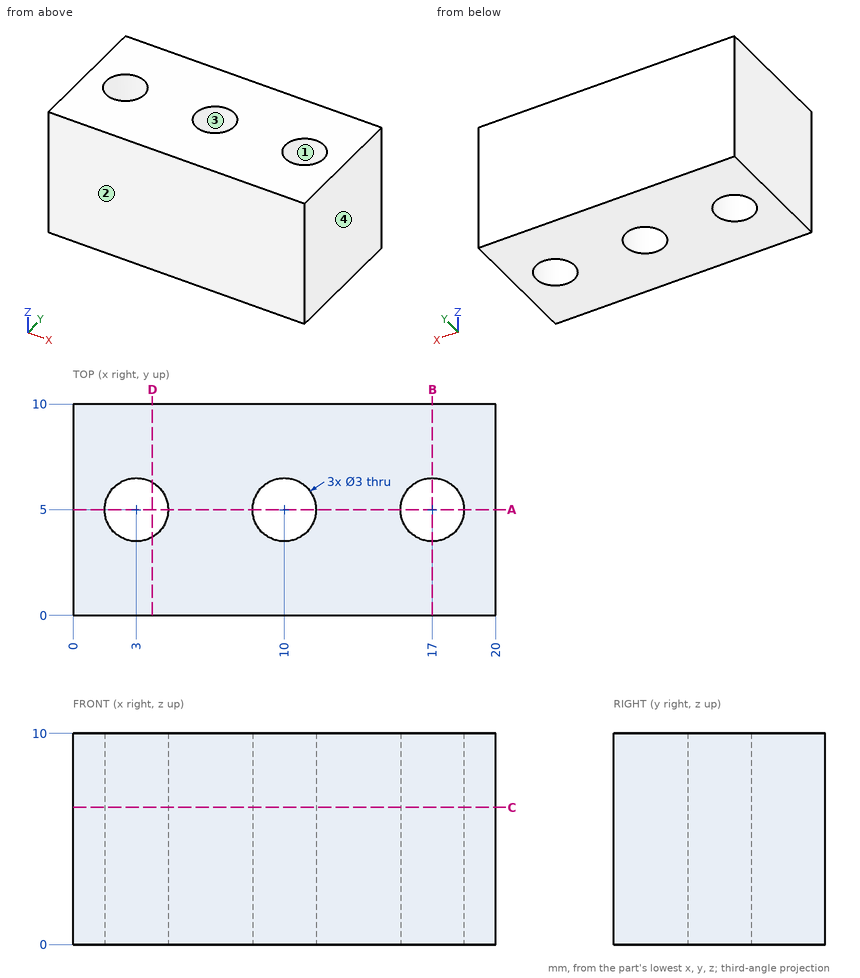
Print and shaded views of the part. All mm, measured from the part's lowest x, y and z. Give positions to 0.01 mm unless a question says otherwise; leave off trailing zeros. Order: outer loops, then holes, each group sorted by start corner. A loop starts at its lowest first (then second) coordinate and runs counter-clockwise, first axis right, second up. Notation, with made-up numbers: (71, 42) - (89, 42) arc R5 ccw to (89, 48) - close; hole circle Ø2 at (-29.75, -4.75). An arc over 180 degrees is marked (long way). Use a Markdown table: item, result.
1) Flat gauge pin, fed straight in: P1, Ø2.5, axis at x = 10, y = 5, coming from the +Z side. Where does the tip first touch, or does it go through?
Checked values:
| item | result |
|---|---|
| P1 | through |
2) Saw through at C-C on z = 6.5. List the corners of the cut face in (x, y), plus the area to 3 significant figures.
Checked values:
| item | result |
|---|---|
| outline | (0, 0) - (20, 0) - (20, 10) - (0, 10) - close; hole circle Ø3 at (3, 5); hole circle Ø3 at (10, 5); hole circle Ø3 at (17, 5) |
| area | 179 mm² |
3) Saw through at A-A on y = 5. List the corners of the cut face in (x, z), plus the area to 3 significant figures.
Checked values:
| item | result |
|---|---|
| outline | (0, 0) - (1.5, 0) - (1.5, 10) - (0, 10) - close; (4.5, 0) - (8.5, 0) - (8.5, 10) - (4.5, 10) - close; (11.5, 0) - (15.5, 0) - (15.5, 10) - (11.5, 10) - close; (18.5, 0) - (20, 0) - (20, 10) - (18.5, 10) - close |
| area | 110 mm² |
4) Two-plate mould, pull along Y, no slides. Class the marked faces 1, 2, 3 and 4: +Y half, -Y half, draft (parallel to the pull), parting line (faces both ways), or undercut.
Checked values:
| item | result |
|---|---|
| face 1 | undercut |
| face 2 | -Y half |
| face 3 | undercut |
| face 4 | draft |
5) Saw through at B-B on x = 17. List the corners of the cut face in (y, z), plus the area to 3 significant figures.
Checked values:
| item | result |
|---|---|
| outline | (0, 0) - (3.5, 0) - (3.5, 10) - (0, 10) - close; (6.5, 0) - (10, 0) - (10, 10) - (6.5, 10) - close |
| area | 70.0 mm² |
6) Saw through at D-D on x = 3.75. List the corners of the cut face in (y, z).
Checked values:
| item | result |
|---|---|
| outline | (0, 0) - (3.7, 0) - (3.7, 10) - (0, 10) - close; (6.3, 0) - (10, 0) - (10, 10) - (6.3, 10) - close |
7) Probe L1, parallel to X at y = 5, z = 7; L2, parallel to Y at x = 10, z = 2; L3, parallel to X at y = 6, z = 9.75. List the from-to ranges inside material, lowest first. Write a range as from..to.
Checked values:
| item | result |
|---|---|
| L1 | 0..1.5, 4.5..8.5, 11.5..15.5, 18.5..20 |
| L2 | 0..3.5, 6.5..10 |
| L3 | 0..1.88, 4.12..8.88, 11.12..15.88, 18.12..20 |
